Geometry check sheet. Reference: the model listing, model coordinates, mm. A direction names the side the tool comes from. Coordinates: 2 decimals unless noted, no trailing zeros. Order: outer loops, then holes, each group sorted by start corner. A loop starts at its lowest first (then second) coordinate and runs counter-clockwise, first axis right, second up. Notation, with made-up numbers: (4, 89.25) - (15, 89.25) arc R32 cw to (15, 121.25) - close; hole circle Ø3 at (42, -8.5). An arc over 180 degrees is marked (long way). Return JSON: item names as keys, results as strings. Group by question number.
Item 1: Section check A-A on z = -218. Enter the section's corners in (x, y), then the cut area to 3 significant figures.
Item 2: Tool access check on faces 1 (the flat face through (-300, -183, 55)), 2 (the flat face through (-193.34, -88.74, 345.84)), 3 (the flat face through (100, -183, -162)). Record the directions out of +Z, -Z, +X, -X, +Y, -Y that give a thin tool (end or side, any length) a straight path to the whole face; none if there is none.
Item 3: Section check B-B on y = -255.5. Enter the section's corners in (x, z), then the cut area to 3 significant figures.
Item 4: Section check C-C on z = 337.5. Enter the section's corners in (x, y).
Item 5: Scan lines: probe 1 along X at (y, z) = (-334, -256); probe 2 along Z at (x, y) = (-17, -69.5); probe 3 along Z at (x, y) = (-104, -194). Record each from-to range of solid material in increasing order.
Item 6: Section check D-D on x = 172.5. Enter the section's corners in (y, z).
Item 7: Gauge pin test, flat ends, axial feed: pin 1 (1.5 mm diameter, centred on x = -29.5, y = -224.5, fed in from +Z); pin 2 (10 mm diameter, centred on x = 5.5, y = -153, fed in from -Z). Record the tip position at first contact, or that the pin passes through.
Item 8: Draft check along Z on faces 4 (the flat face through (300, -183, 55)), 5 (the flat face through (-1, -183, -35)), 6 (the flat face through (-4, -217, 285)). Enter one of: pulls with the +Z half, pulls with the -Z half, needs draft (parallel to the pull), parting line crosses it, or undercut.
from build123d import *

# Parameters (mm, degrees)
F0_W      = 600
F0_H      = 570
F1_DEPTH  = 360
F2_W      = 200
F2_H      = 250
F3_DEPTH  = 500
F4_W      = 210.372046
F4_H      = 180
F5_DEPTH  = 120
F7_DEPTH  = 120
F8_W      = 184.683776
F8_H      = 180
F9_DEPTH  = 120
F11_DEPTH = 120


with BuildPart() as f1:
    # F0 (on Front) → F1 (new body)
    with BuildSketch(Plane.XZ):
        Rectangle(F0_W, F0_H)
    extrude(amount=F1_DEPTH)

    # F2 (on face) → F3 (cut)
    with BuildSketch(Plane.XZ.offset(360)):
        with Locations((0, -160)):
            Rectangle(F2_W, F2_H)
    extrude(amount=-F3_DEPTH, mode=Mode.SUBTRACT)

    # F4 (on face) → F5 (join)
    with BuildSketch(Plane.XY.offset(285)):
        with Locations((-194.813977, -90)):
            Rectangle(F4_W, F4_H)
    extrude(amount=F5_DEPTH)

    # F6 (on face) → F7 (cut)
    with BuildSketch(Plane.XY.offset(405)):
        Polygon((-89.627954, -180), (-89.627954, 0), (-300, -180), align=None)
    extrude(amount=-F7_DEPTH, mode=Mode.SUBTRACT)

    # F8 (on face) → F9 (join)
    with BuildSketch(Plane.XY.offset(285)):
        with Locations((207.658112, -90)):
            Rectangle(F8_W, F8_H)
    extrude(amount=F9_DEPTH)

    # F10 (on face) → F11 (cut)
    with BuildSketch(Plane.XY.offset(405)):
        Polygon((300, -180), (115.316224, 0), (115.316224, -180), align=None)
    extrude(amount=-F11_DEPTH, mode=Mode.SUBTRACT)


solid = f1.part
Computed:
{
 "1": {"outline": "(-300, -360) - (-100, -360) - (-100, 0) - (-300, 0) - close; (100, -360) - (300, -360) - (300, 0) - (100, 0) - close", "area": "144,000 mm²"},
 "2": {"face 1": "+Z, -Z, -X, +Y, -Y", "face 2": "+Z, -Y", "face 3": "-Z, +Y, -Y"},
 "3": {"outline": "(-300, -285) - (-100, -285) - (-100, -35) - (100, -35) - (100, -285) - (300, -285) - (300, 285) - (-300, 285) - close", "area": "292,000 mm²"},
 "4": {"outline": "(-300, -180) - (-89.63, 0) - (-300, 0) - close; (115.32, 0) - (300, -180) - (300, 0) - close"},
 "5": {"probe 1": "x = -300 to -100, 100 to 300", "probe 2": "z = -35 to 285", "probe 3": "z = -285 to 285"},
 "6": {"outline": "(-360, -285) - (0, -285) - (0, 405) - (-55.73, 405) - (-55.73, 285) - (-360, 285) - close"},
 "7": {"pin 1": "stops at z = 285", "pin 2": "stops at z = -35"},
 "8": {"face 4": "needs draft", "face 5": "pulls with the -Z half", "face 6": "pulls with the +Z half"}
}
